Geometry check sheet. Reference: the model listing, model coordinates, mm. Face numbers are marked on the shaded views. Give positions to 0.01 mm unless a question says otherwise; leave off trailing zeros. Write each loop counter-clockwise with the first axis right and the second up, starting at its lowest first coordinate (ties: lowest second). Pieces come first, ordered by that corner, then holes. Notation, with made-up numbers: (87, 58.25) - (109, 58.25) arc R19 cw to (109, 71.25) - close; hole circle Ø7 at (-32.5, 38.25). An arc over 180 degrees is marked (long way). One line per question, with ' | ' between items. Start each with the question number.
Q1. Section check C-C on y = -6. Record the boundary of the cut face in (x, z), and give its area (3 significant figures).
Q2. Release check for a two-part mould opening along Z. For the marked faces 1, 2 and 3 record: +Z half, -Z half, draft (parallel to the pull), parting line (faces both ways), or undercut.
Q3. Gauge pin test, flat ends, axial feed: P1, Ø1, axis at x = -15.5, y = -0.5, coming from the +Z side; P2, Ø4, axis at y = 2, z = 13, coming from the +X side; P3, Ø2, axis at y = -3, z = -8.5, coming from the +X side; P4, Ø10, axis at x = -17, z = 11, coming from the +Y side. Record the tip position at first contact, or that the pin passes through.
Q4. Section check D-D on y = 1. Record the boundary of the cut face in (x, z).
Q5. Thickness scan on L1, parallel to X at y = -4, z = 0; L2, parallel to X at y = 1.8, z = 0; L3, parallel to Z at x = -8.5, y = -4.5. Record the ranges inside material, lowest first. Write a range as [from, to].
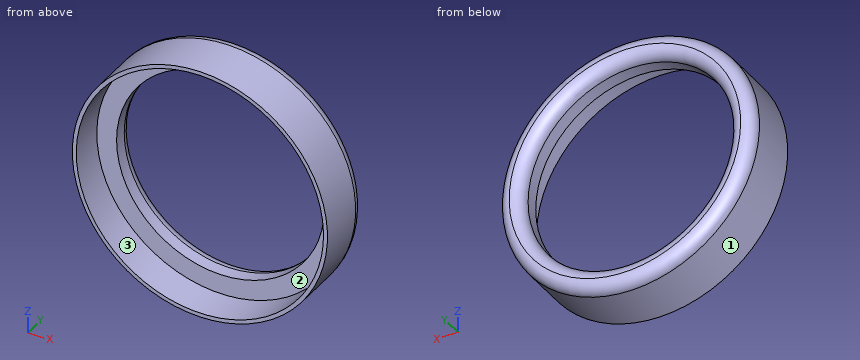
```python
from build123d import *

# Parameters (mm, degrees)
SKETCH1_R           = 25.8
SKETCH1_R_2         = 25
BOSS_EXTRUDE1_DEPTH = 7
BOSS_EXTRUDE2_START = 5
SKETCH2_R           = 25.8
SKETCH2_R_2         = 21
BOSS_EXTRUDE2_DEPTH = 5
FILLET3_R           = 2.4


with BuildPart() as part:
    # Sketch1 → Boss-Extrude1 (new body)
    with BuildSketch(Plane(origin=(0, 0, 0), x_dir=(1, 0, 0), z_dir=(0, 1, 0))):
        with Locations(Location((0, 0, 0), (0, 0, 270))):
            Circle(SKETCH1_R)
        with Locations(Location((0, 0, 0), (0, 0, 270))):
            Circle(SKETCH1_R_2, mode=Mode.SUBTRACT)
    extrude(amount=-BOSS_EXTRUDE1_DEPTH)

    # Sketch2 → Boss-Extrude2 (add)
    with BuildSketch(Plane(origin=(0, 0, 0), x_dir=(1, 0, 0), z_dir=(0, 1, 0)).offset(BOSS_EXTRUDE2_START)):
        with Locations(Location((0, 0, 0), (0, 0, 270))):
            Circle(SKETCH2_R)
        with Locations(Location((0, 0, 0), (0, 0, 270))):
            Circle(SKETCH2_R_2, mode=Mode.SUBTRACT)
    extrude(amount=-BOSS_EXTRUDE2_DEPTH)

    # Fillet3
    fillet3_edges = [part.edges().sort_by_distance(p)[0] for p in [
        (0, 5, -25.8),
        (0, 5, -21),
    ]]
    fillet(fillet3_edges, radius=FILLET3_R - 0.0001)  # a hair under: the kernel refuses the full size


solid = part.part
```
Working result:
1) outline: circle Ø51.6 at (0, 0); hole circle Ø50 at (0, 0) | area: 128 mm2
2) face 1: parting line | face 2: undercut | face 3: undercut
3) P1: stops at z = 20.99 | P2: stops at x = 23.34 | P3: stops at x = 24.69 | P4: stops at y = 5
4) outline: circle Ø51.6 at (0, 0); hole circle Ø42 at (0, 0)
5) L1: x = [-25.8, -25], [25, 25.8] | L2: x = [-25.8, -21], [21, 25.8] | L3: z = [-24.36, -23.51], [23.51, 24.36]
